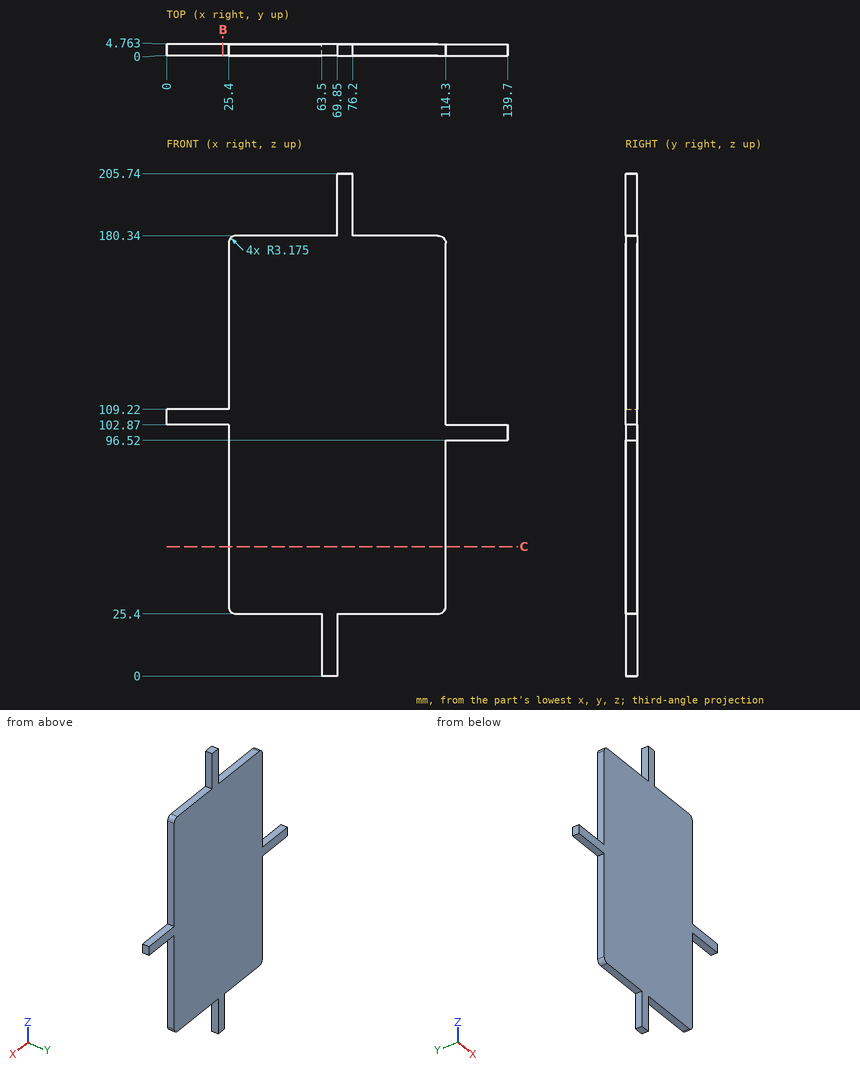
For this review, use the dimensioned drawing (mm, ordinates from the lowest corner) and the shaded views. Round coordinates to 2 decimals unless told otherwise and drop trailing zeros. Write each loop counter-clockwise with the first axis right and the second up, starting at its lowest first coordinate (ties: lowest second). Pieces come first, ordered by that corner, then holes. Notation, with made-up numbers: (62, 0) -> (103, 0) arc R20 ccw to (103, 10) -> close; hole circle Ø3 at (-35, 10). An arc over 180 degrees is marked (long way). One line per item, written item: value. Start each with the question number.
Q1. To check wall thickness, follow probe 1 along Z at (x, y) = (96.5, 3.75); probe 2 along X at (y, z) = (2.95, 71); probe 3 along X at (y, z) = (4.4, 9). State the ranges of each line that lie inside material, in increasing order.
Q2. Insertion check: P1, Ø2.5, axis at x = 133, y = 1.5, coming from the -Z side; P2, Ø2.5, axis at y = 3.5, z = 194.5, coming from the -X side; P3, Ø1.4, axis at y = 2.5, z = 18, coming from the -X side. Each pin has a flat end and moves straight along its axis. Give the tip position at first contact, or say it passes through.
Q3. Add section B-B (x = 23). Give the boundary of the cut face in (y, z).
Q4. Add section C-C (z = 53). Give the boundary of the cut face in (x, y).
Response:
1. probe 1: z = 25.4 to 180.34
1. probe 2: x = 25.4 to 114.3
1. probe 3: x = 63.5 to 69.85
2. P1: stops at z = 96.52
2. P2: stops at x = 69.85
2. P3: stops at x = 63.5
3. outline: (0, 102.87) -> (4.76, 102.87) -> (4.76, 109.22) -> (0, 109.22) -> close
4. outline: (25.4, 0) -> (114.3, 0) -> (114.3, 4.76) -> (25.4, 4.76) -> close
